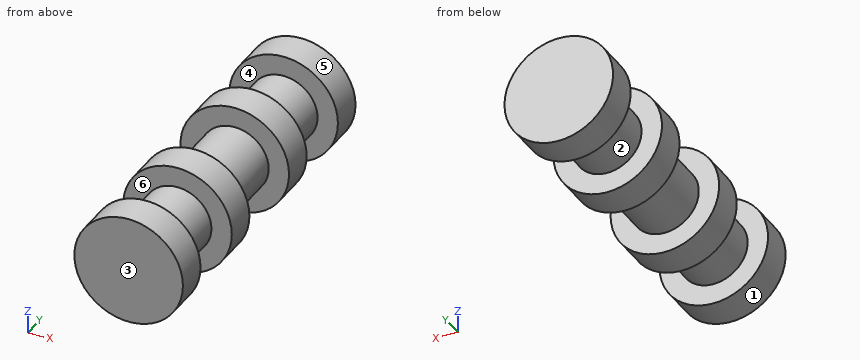
Autodesk Inventor part; units mm, degrees
ref_plane "YZ Plane" through (0, 0, 0) normal (1, 0, 0) x (0, 1, 0)
ref_plane "XZ Plane" through (0, 0, 0) normal (0, 1, 0) x (-1, 0, 0)
ref_plane "XY Plane" through (0, 0, 0) normal (0, 0, 1) x (1, 0, 0)
sketch "Sketch1" plane through (0, 0, 0) normal (0, 0, 1) x (1, 0, 0)
  line L0 (0, 0) -> (0, 31.115)
  line L1 (0, 31.115) -> (5.08, 31.115)
  line L2 (5.08, 31.115) -> (5.08, 27.94)
  line L3 (5.08, 27.94) -> (3.175, 27.94)
  line L4 (3.175, 15.5575) -> (3.175, 19.1294)
  line L5 (3.175, 19.1294) -> (5.08, 19.1294)
  line L6 (5.08, 19.1294) -> (5.08, 22.3044)
  line L7 (5.08, 22.3044) -> (3.175, 22.3044)
  line L8 (3.175, 15.5575) -> (3.175, 19.1294)
  line L9 (3.175, 22.3044) -> (3.175, 27.94)
  line L10 (0, 0) -> (5.08, 0)
  line L11 (5.08, 0) -> (5.08, 3.175)
  line L12 (5.08, 3.175) -> (3.175, 3.175)
  line L13 (3.175, 15.5575) -> (3.175, 11.9856)
  line L14 (3.175, 11.9856) -> (5.08, 11.9856)
  line L15 (5.08, 11.9856) -> (5.08, 8.8106)
  line L16 (5.08, 8.8106) -> (3.175, 8.8106)
  line L17 (3.175, 15.5575) -> (3.175, 11.9856)
  line L18 (3.175, 8.8106) -> (3.175, 3.175)
  dimension "d0" = 31.115
  dimension "d1" = 5.08
  dimension "d2" = 3.175
  dimension "d5" = 3.175
revolve "Revolution1" add sketch "Sketch1" angle 360 about axis through (0, 0, 0) along (0, 1, 0)
properties part number "Wrist Pin"
For this review, take the finished solid that the model builds, in its own axes (mm). Face numbers are marked on the shaded views. A direction names the side the tool comes from. Give positions to 0.01 mm unless a question says otherwise; leave off trailing zeros. Order: outer loops, then holes, each group sorted by start corner. A loop starts at its lowest first (then second) coordinate and runs counter-clockwise, first axis right, second up. Notation, with made-up numbers: (24, 20.5) - (44, 20.5) arc R24 cw to (44, 46.5) - close; hole circle Ø6 at (13, 83.25). An arc over 180 degrees is marked (long way). Answer as a JSON object with one key per item and string values. Group by question number.
Item 1: Wall thickness on line 1 along Y through (x, z) = (3, -2.25) (3 decimals); line 2 along X through (y, z) = (18.5, -0.5); line 3 along Z through (x, y) = (1.75, 16.5): over which ranges is each line inside the solid? List them lowest first.
Item 2: Take a section at A-A on x = 3.5. Give the boundary of the cut face in (y, z) (3 decimals).
Item 3: Clearance check with flat-ended pins moving along their axes: pin 1 Ø2 at (y, z) = (20, 3) entering from +X; pin 2 Ø1.5 at (y, z) = (22.5, -3.5) entering from -X; pin 3 Ø1.5 at (x, y) = (0.5, 25.5) entering from +Z (3 decimals). State where each tip first meets the part, or that it passes through.
Item 4: Machinability: for the marked faces 1 and 2, which of the approach directions +Z, -Z, +X, -X, +Y, -Y give a long, thin tool a straight path to every point of the face, cutting with its end or side? Answer none if there is none.
Item 5: Take a section at B-B on z = 0. Give the boundary of the cut face in (x, y) (3 decimals).
Item 6: Take a section at D-D on y = 26.5. Give the boundary of the cut face in (x, z) (3 decimals).
Item 7: Draft analysis for pull direction Y (two halves, no side actions). For the marked faces 3, 4, 5 and 6, state which applies: pulls with the +Y half, pulls with the -Y half, needs draft (parallel to the pull), parting line crosses it, or undercut.
Item 8: Take a section at C-C on x = 0. Give the boundary of the cut face in (y, z) (3 decimals), and give its area (3 significant figures).
Reported:
{
 "1": {"line 1": "0 to 3.175, 8.811 to 11.986, 19.129 to 22.304, 27.94 to 31.115", "line 2": "-3.14 to 3.14", "line 3": "-2.65 to 2.65"},
 "2": {"outline": "(0, -3.682) - (3.175, -3.682) - (3.175, 3.682) - (0, 3.682) - close; (8.811, -3.682) - (11.986, -3.682) - (11.986, 3.682) - (8.811, 3.682) - close; (19.129, -3.682) - (22.304, -3.682) - (22.304, 3.682) - (19.129, 3.682) - close; (27.94, -3.682) - (31.115, -3.682) - (31.115, 3.682) - (27.94, 3.682) - close"},
 "3": {"pin 1": "x = 4.67", "pin 2": "x = -4.25", "pin 3": "z = 3.175"},
 "4": {"face 1": "+Y, -Y", "face 2": "none"},
 "5": {"outline": "(-5.08, 0) - (5.08, 0) - (5.08, 3.175) - (3.175, 3.175) - (3.175, 8.811) - (5.08, 8.811) - (5.08, 11.986) - (3.175, 11.986) - (3.175, 19.129) - (5.08, 19.129) - (5.08, 22.304) - (3.175, 22.304) - (3.175, 27.94) - (5.08, 27.94) - (5.08, 31.115) - (-5.08, 31.115) - (-5.08, 27.94) - (-3.175, 27.94) - (-3.175, 22.304) - (-5.08, 22.304) - (-5.08, 19.129) - (-3.175, 19.129) - (-3.175, 11.986) - (-5.08, 11.986) - (-5.08, 8.811) - (-3.175, 8.811) - (-3.175, 3.175) - (-5.08, 3.175) - close"},
 "6": {"outline": "circle Ø6.35 at (0, 0)"},
 "7": {"face 3": "pulls with the -Y half", "face 4": "undercut", "face 5": "needs draft", "face 6": "undercut"},
 "8": {"outline": "(0, -5.08) - (3.175, -5.08) - (3.175, -3.175) - (8.811, -3.175) - (8.811, -5.08) - (11.986, -5.08) - (11.986, -3.175) - (19.129, -3.175) - (19.129, -5.08) - (22.304, -5.08) - (22.304, -3.175) - (27.94, -3.175) - (27.94, -5.08) - (31.115, -5.08) - (31.115, 5.08) - (27.94, 5.08) - (27.94, 3.175) - (22.304, 3.175) - (22.304, 5.08) - (19.129, 5.08) - (19.129, 3.175) - (11.986, 3.175) - (11.986, 5.08) - (8.811, 5.08) - (8.811, 3.175) - (3.175, 3.175) - (3.175, 5.08) - (0, 5.08) - close", "area": "246 mm^2"}
}
